For this review, take the finished solid that the model builds, in its own axes (mm). Coordinates: 2 decimals unless noted, no trailing zeros. Write each loop counter-clockwise with the first axis right and the second up, starting at its lowest first coordinate (ties: lowest second). Pieces come first, ordered by that corner, then holes.
1) We need section D-D on x = -56.5. Write out the cut boundary in (y, z), then the cut area to 3 significant figures.
2) We need section C-C on x = -4. Write out the cut boundary in (y, z).
3) We need section A-A on x = 74. Write out the cut boundary in (y, z).
4) To check wall thickness, follow line 1 along Y through (x, z) = (-73.4, 2.2); line 2 along X through (y, z) = (-8, 2.45); line 3 along Y through (x, z) = (90.5, 2.05). State the ranges of each line that lie inside material, in increasing order.
5) We need section B-B on z = 1.95. Give the number of separate pieces and of enclosed holes in the cut face, then the cut area to 3 significant figures.
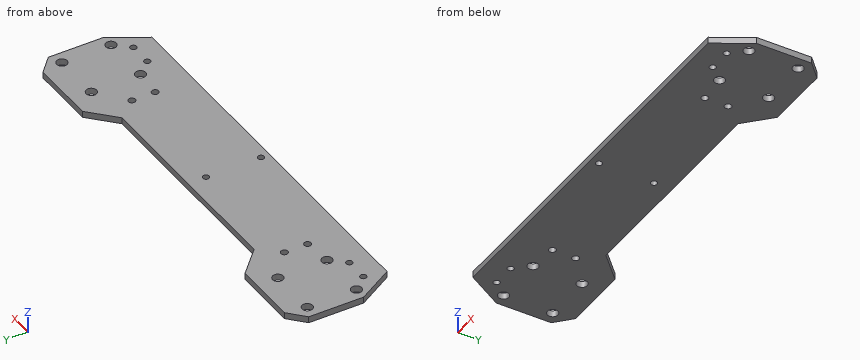
from build123d import *

# Parameters (mm, degrees)
SKETCH_R     = 2.5
SKETCH_R_2   = 1.5
SKETCH_R_3   = 1.65
PAD_DEPTH    = 3
SKETCH001_R  = 1.5
POCKET_DEPTH = 3.001


with BuildPart() as part:
    # Sketch → Pad (new body)
    with BuildSketch(Plane.XY):
        Polygon((0, -11.5), (-52, -11.5), (-64, 0), (-95, 0), (-102.5, -7), (-102.5, -33), (-92.5, -50), (0, -50), align=None)
        with Locations((-96.6, -9.9)):
            Circle(SKETCH_R, mode=Mode.SUBTRACT)
        with Locations((-73.4, -9.9)):
            Circle(SKETCH_R, mode=Mode.SUBTRACT)
        with Locations((-73.4, -33.1)):
            Circle(SKETCH_R, mode=Mode.SUBTRACT)
        with Locations((-96.6, -33.1)):
            Circle(SKETCH_R, mode=Mode.SUBTRACT)
        with Locations((-90.5, -40)):
            Circle(SKETCH_R_2, mode=Mode.SUBTRACT)
        with Locations((-79.5, -40)):
            Circle(SKETCH_R_2, mode=Mode.SUBTRACT)
        with Locations((-60, -21)):
            Circle(SKETCH_R_3, mode=Mode.SUBTRACT)
        with Locations((-60, -32)):
            Circle(SKETCH_R_3, mode=Mode.SUBTRACT)
    pad = extrude(amount=PAD_DEPTH)

    # Mirrored: Pad across Sketch V_Axis
    add(pad.mirror(Plane(origin=(0, 0, 0), x_dir=(0, 0, 1), z_dir=(1, 0, 0))))

    # Sketch001 → Pocket (cut, through all)
    with BuildSketch(Plane.XY.offset(3)):
        with Locations((0, -20)):
            Circle(SKETCH001_R)
        with Locations((0, -46)):
            Circle(SKETCH001_R)
    extrude(amount=-POCKET_DEPTH, mode=Mode.SUBTRACT)


solid = part.part
Result:
1. outline: (-50, 0) - (-7.19, 0) - (-7.19, 3) - (-50, 3) - close
1. area: 128 mm2
2. outline: (-50, 0) - (-11.5, 0) - (-11.5, 3) - (-50, 3) - close
3. outline: (-50, 0) - (-35.53, 0) - (-35.53, 3) - (-50, 3) - close; (-30.67, 0) - (-12.33, 0) - (-12.33, 3) - (-30.67, 3) - close; (-7.47, 0) - (0, 0) - (0, 3) - (-7.47, 3) - close
4. line 1: y = -50 to -35.6, -30.6 to -12.4, -7.4 to 0
4. line 2: x = -102.5 to -98.22, -94.98 to -75.02, -71.78 to -55.65, 55.65 to 71.78, 75.02 to 94.98, 98.22 to 102.5
4. line 3: y = -50 to -41.5, -38.5 to 0
5. separate pieces: 1
5. enclosed holes: 18
5. area: 8,460 mm2
